Answer from the drawing. Dimensions are ordinates in mm from the lowest x, y and z of the part. Coordinates: 2 decimals unless noted, no trailing zeros. Order: outer loops, then holes, each group sorted by start corner. A loop starts at its lowest first (then second) coordinate and runs counter-clockwise, first axis right, second up. Notation, with made-up numbers: (-23, 6.5) -> (-11, 6.5) arc R22 ccw to (-11, 36.5) -> close; hole circle Ø4 at (68, 87). An arc over 180 degrees is marked (long way). Answer in a Markdown table with one row per item.
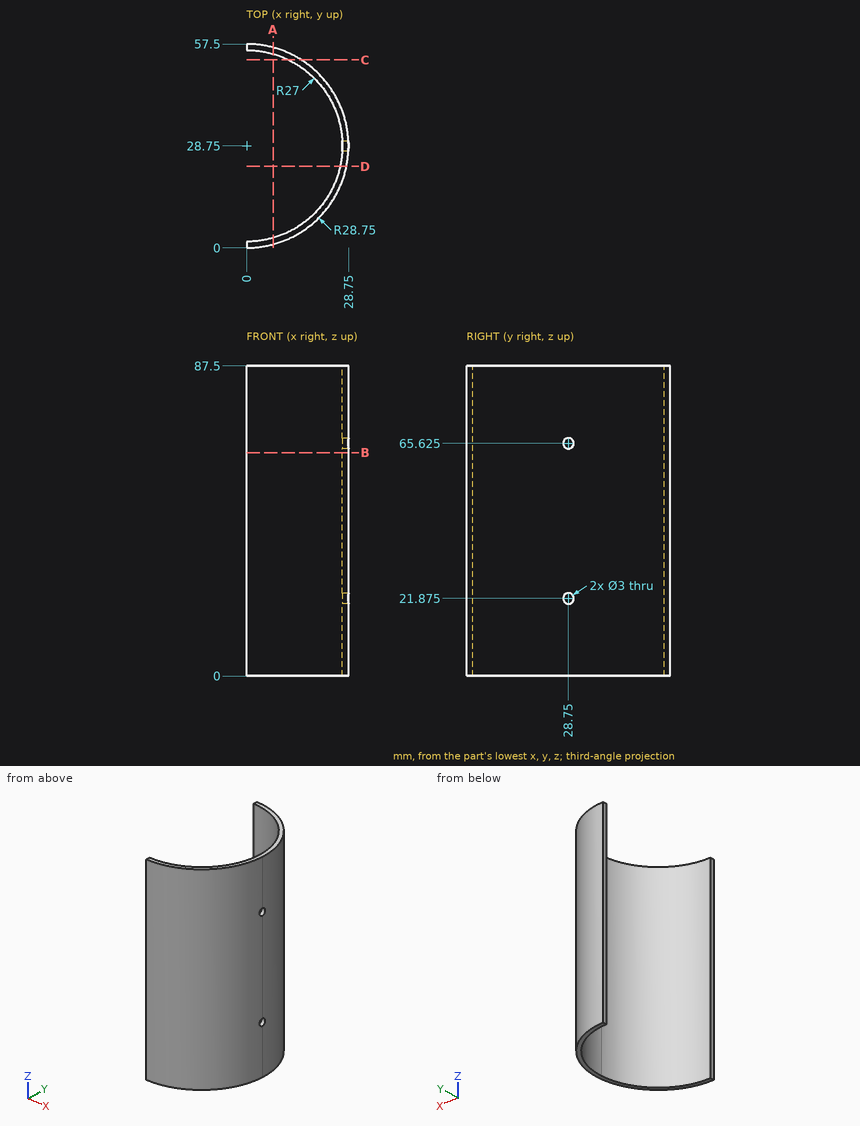
Q1. The part is cut by section B-B (z = 63). Write down the section's boundary in (x, y), then the cut area to 3 significant figures.
Outcome:
| item | result |
|---|---|
| outline | (0, 0) arc R28.75 ccw to (0, 57.5) -> (0, 55.75) arc R27 cw to (0, 1.75) -> close |
| area | 153 mm² |
Q2. Consider line 1 (Y direction, x = 1.5, z = 68.5); line 2 (Y direction, x = 24.5, z = 52); line 3 (X direction, y = 26, z = 60). Determine where each line is inside the solid, lowest interval first.
Outcome:
| item | result |
|---|---|
| line 1 | 0.04 to 1.79, 55.71 to 57.46 |
| line 2 | 13.71 to 17.4, 40.1 to 43.79 |
| line 3 | 26.86 to 28.62 |
Q3. Given pin 1 (3 mm diameter, centred on y = 51, z = 66.5, fed in from -X); pin 2 (10 mm diameter, centred on x = 13.5, y = 42.5, fed in from -Z); pin 3 (1.5 mm diameter, centred on y = 28, z = 55.5, fed in from -X); pin 4 (4 mm diameter, centred on x = 25.5, z = 53.5, fed in from -Y), each flat-ended and moving along its own axis, determine where each tip first touches the part or whether it passes through.
Outcome:
| item | result |
|---|---|
| pin 1 | x = 12.84 |
| pin 2 | through |
| pin 3 | x = 26.96 |
| pin 4 | y = 12.19 |
Q4. The part is cut by section C-C (y = 53). Write down the section's boundary in (x, z).
Outcome:
| item | result |
|---|---|
| outline | (11.87, 0) -> (15.44, 0) -> (15.44, 87.5) -> (11.87, 87.5) -> close |
Q5. The part is cut by section D-D (y = 23). Write down the section's boundary in (x, z).
Outcome:
| item | result |
|---|---|
| outline | (26.38, 0) -> (28.17, 0) -> (28.17, 87.5) -> (26.38, 87.5) -> close |
Q6. The part is cut by section A-A (x = 7.5). Write down the section's boundary in (y, z).
Outcome:
| item | result |
|---|---|
| outline | (1, 0) -> (2.81, 0) -> (2.81, 87.5) -> (1, 87.5) -> close; (54.69, 0) -> (56.5, 0) -> (56.5, 87.5) -> (54.69, 87.5) -> close |
